Autodesk Fusion 360 part; units mm, degrees
sketch "Sketch1" plane through (0, 0, 0) normal (0, 1, 0) x (1, 0, 0)
  line L0 (-29.5, 50) -> (50, 50)
  line L1 (50, 50) -> (50, 0)
  line L2 (50, 0) -> (-29.5, 0)
  line L3 (-29.5, 0) -> (-29.5, 50)
  line L4 (54, -4) -> (-33.5, -4)
  line L5 (-33.5, -4) -> (-33.5, 54)
  line L6 (-33.5, 54) -> (54, 54)
  line L7 (54, 54) -> (54, -4)
  line L8 (47, 3) -> (-26.5, 3)
  line L9 (-26.5, 3) -> (-26.5, 47)
  line L10 (-26.5, 47) -> (47, 47)
  line L11 (47, 47) -> (47, 3)
  dimension "d1" = 50
  dimension "d2" = 79.5
  dimension "d3" = -4
  dimension "d6" = 3
extrude "Extrude1" add sketch "Sketch1" along normal blind 5 contours L4 L5 L6 L7 makes body 1
extrude "Extrude2" add sketch "Sketch1" along normal blind 5 separate body contours L0 L1 L2 L3 makes body 2
sketch "Sketch2" plane through (0, 5, 0) normal (0, 1, 0) x (-1, 0, 0)
  line L0 (-50, 0) -> (29.5, 0)
  line L1 (29.5, 0) -> (29.5, -50)
  line L2 (29.5, -50) -> (-50, -50)
  line L3 (-50, -50) -> (-50, 0)
  line L4 (-54, -54) -> (33.5, -54)
  line L5 (33.5, -54) -> (33.5, 4)
  line L6 (33.5, 4) -> (-54, 4)
  line L7 (-54, 4) -> (-54, -54)
  line L8 (-10.25, -54) -> (-10.25, 4)
extrude "Extrude3" add sketch "Sketch2" along normal blind 10 contours L0 L2 L3 L4 L6 L7 L8 bodies 1 2
sketch "Sketch3" plane through (0, 5, 0) normal (0, 1, 0) x (-1, 0, 0)
  line L0 (-10.25, 4) -> (-10.25, 0)
  line L1 (-10.25, 0) -> (-50, 0)
  line L2 (-50, 0) -> (-50, -50)
  line L3 (-50, -50) -> (-10.25, -50)
  line L4 (-10.25, -50) -> (-10.25, -54)
  line L5 (-10.25, -54) -> (33.5, -54)
  line L6 (33.5, -54) -> (33.5, 4)
  line L7 (33.5, 4) -> (-10.25, 4)
  line L8 (26.5, -47) -> (-47, -47)
  line L9 (-47, -47) -> (-47, -3)
  line L10 (-47, -3) -> (26.5, -3)
  line L11 (26.5, -3) -> (26.5, -47)
  line L12 (-50, 0) -> (-50, -0.25)
  line L13 (-50, -0.25) -> (29, -0.25)
  line L14 (29, -0.25) -> (29, -49.75)
  line L15 (29, -49.75) -> (-50, -49.75)
  line L16 (-49.75, -79.25) -> (-49.75, -0.25)
  dimension "d11" = 0.25
  dimension "d12" = 49.5
Geometry check sheet. Reference: the model listing, model coordinates, mm. A direction names the side the tool comes from. Give positions to 0.01 mm unless a question says otherwise; leave off trailing zeros. Write each loop counter-clockwise with the first axis right and the second up, starting at its lowest first coordinate (ties: lowest second). Pieces come first, ordered by that corner, then holes. Notation, with made-up numbers: M 84.5,-2 L 123.5,-2 A19 ccw 123.5,25 Z; hole C 44.5,-39 d3. An arc over 180 degrees is marked long. Answer as CSV lines item,"result". Start each with the question number.
Q1. Go/stop test with flat-tipped pins: pin 1 (3 mm diameter, centred on x = -24, z = -39, fed in from +Y); pin 2 (4.5 mm diameter, centred on y = 8, z = 2.5, fed in from -X); pin 3 (2 mm diameter, centred on y = 9.5, z = -19.5, fed in from -X). Record where each tip stops, or that it passes through.
Q2. Section check C-C, the plane y = 2. Record the cut outline in (x, z).
Q3. Material ranges on L1, parallel to Z at x = 37, y = 8.25; L2, parallel to Z at x = -6, y = 3.25; L3, parallel to X at y = 1.75, z = -30, recorded low to high.
Q4. Section check D-D, the plane x = 41. Record the cut outline in (y, z), then the cut area to 3 significant figures.
Q5. Release check for a two-part mould opening along X. For faces 5 (the face through (-33.5, 2, -25)), 6 (the face through (47, 2, -25)), 7 (the face through (-26.5, 2, -25)), 8 (the face through (30, 10, -50)) record: pulls with the +X half, pulls with the -X half, needs draft (parallel to the pull), parting line crosses it, or undercut.
Q6. Section check A-A, the plane x = -15. Record the cut outline in (y, z), then the cut area to 3 significant figures.
Q7. Section check B-B, the plane z = -20.5. Record the cut outline in (x, y).
Q8. Tool access check on faces 1 (the face through (10, 0, 0)), 2 (the face through (30, 10, 0)), 3 (the face through (10.25, 10, 2)), 4 (the face through (10, 2, -47)). Record the directions out of +Z, -Z, +X, -X, +Y, -Y that give a thin tool (end or side, any length) a straight path to the whole face; none if there is none.
Geometry says:
1,pin 1,"through"
1,pin 2,"x = 10.25"
1,pin 3,"x = 50"
2,outline,"M -33.5,-54 L 54,-54 L 54,4 L -33.5,4 Z; hole M -26.5,-47 L 47,-47 L 47,-3 L -26.5,-3 Z"
3,L1,"-54 to -50, 0 to 4"
3,L2,"-54 to -47, -3 to 4"
3,L3,"-33.5 to -26.5, 47 to 54"
4,outline,"M 0,-54 L 15,-54 L 15,-50 L 5,-50 L 5,-47 L 0,-47 Z; M 0,-3 L 5,-3 L 5,0 L 15,0 L 15,4 L 0,4 Z"
4,area,"150 mm^2"
5,face 5,"pulls with the -X half"
5,face 6,"undercut"
5,face 7,"undercut"
5,face 8,"needs draft"
6,outline,"M 0,-54 L 5,-54 L 5,-47 L 0,-47 Z; M 0,-3 L 5,-3 L 5,4 L 0,4 Z"
6,area,"70.0 mm^2"
7,outline,"M -33.5,0 L -26.5,0 L -26.5,5 L -33.5,5 Z; M 47,0 L 54,0 L 54,15 L 50,15 L 50,5 L 47,5 Z"
8,face 1,"+Z, -Z, +X, -X, -Y"
8,face 2,"-X, +Y"
8,face 3,"+Z, -Z, -X, +Y"
8,face 4,"+Y, -Y"
